Part model, mm, in its own coordinate system. Face numbers are marked on the shaded views. A direction names the side the tool comes from. Coordinates: 2 decimals unless noted, no trailing zeros. Write each loop counter-clockwise with the first axis right and the second up, starting at its lowest first coordinate (ties: lowest second). Pieces come first, ordered by that corner, then holes. Notation, with made-up numbers: (-25, 25) -> (29, 25) arc R16 cw to (29, 45) -> close; hole circle Ø5 at (57, -5.75). An arc over 180 degrees is marked (long way). One line per question, with ' | ' between items. Start each with the question number.
Item 1: Two-plate mould, pull along Y, no slides. Class the marked faces 1, 2 and 3: pulls with the +Y half, pulls with the -Y half, needs draft (parallel to the pull), parting line crosses it, or undercut.
Item 2: Probe probe 1 along Y at (x, z) = (0, -18); probe 2 along Z at (x, y) = (-20, 8.5). List the from-to ranges inside material, lowest first. Write a range as [from, to].
Item 3: Saw through at C-C (x = -43). List the corners of the cut face in (y, z), and give its area (3 significant figures).
Item 4: Saw through at B-B (y = 18). List the corners of the cut face in (x, z).
Item 5: 3-axis set-ups, long thin cutter, end or side, ignore diameter. For the marked faces 4 and 5: which of +Z, -Z, +X, -X, +Y, -Y reach the whole face in a straight line?
Item 6: Pin check, flat tips, straight feed: pin 1 (2 mm diameter, centred on x = 21.5, y = -9, fed in from -Z); pin 2 (5 mm diameter, centred on x = 0, y = 0, fed in from +Z). Stop position of each tip, or through.
Item 7: Saw through at A-A (z = -12). List the corners of the cut face in (x, y), and give its area (3 significant figures).
from build123d import *

# Parameters (mm, degrees)
F1_DEPTH = 10
F2_R     = 2
F3_DEPTH = 10
F2_R_2   = 4
F4_DEPTH = 5
F5_R     = 4.99999
F6_R     = 5
F6_R_2   = 2
F7_DEPTH = 25


# Not quite as in the source:
# - a fillet or chamfer is up to 0.001 mm smaller than in the source, because OpenCascade refuses the exact size


with BuildPart() as f1:
    # F0 (on Top) → F1 (new body)
    with BuildSketch(Plane.XY):
        with BuildLine():
            ThreePointArc((-50, -5), (-18.1801948466, -18.1801948466), (-5, -50))
            Line((-5, -50), (5, -50))
            ThreePointArc((5, -50), (18.1801948466, -18.1801948466), (50, -5))
            Line((50, -5), (50, 5))
            ThreePointArc((50, 5), (18.1801948466, 18.1801948466), (5, 50))
            Line((5, 50), (-5, 50))
            ThreePointArc((-5, 50), (-18.1801948466, 18.1801948466), (-50, 5))
            Line((-50, 5), (-50, -5))
        make_face()
    extrude(amount=F1_DEPTH)

    # F2 (on face) → F3 (cut, through all)
    with BuildSketch(Plane.XY.offset(10)):
        Circle(F2_R)
    extrude(amount=-F3_DEPTH, mode=Mode.SUBTRACT)

    # F2 (on face) → F4 (cut)
    with BuildSketch(Plane.XY.offset(10)):
        Circle(F2_R_2)
        Circle(F2_R, mode=Mode.SUBTRACT)
    extrude(amount=-F4_DEPTH, mode=Mode.SUBTRACT)

    # F5 (radius 5 in the source; OpenCascade refuses exactly that, so slightly less here)
    f5_edges = [f1.edges().sort_by_distance(p)[0] for p in [
        (5, 50, 5),
        (-5, 50, 5),
        (0, 50, 0),
        (0, 50, 10),
        (-50, 5, 5),
        (-50, -5, 5),
        (-50, 0, 0),
        (-50, 0, 10),
        (-5, -50, 5),
        (5, -50, 5),
        (0, -50, 0),
        (0, -50, 10),
        (50, -5, 5),
        (50, 5, 5),
        (50, 0, 0),
        (50, 0, 10),
    ]]
    fillet(f5_edges, radius=F5_R)

    # F6 (on face) → F7 (join)
    with BuildSketch(Plane(origin=(0, 0, 0), x_dir=(1, 0, 0), z_dir=(0, 0, -1))):
        Circle(F6_R)
        Circle(F6_R_2, mode=Mode.SUBTRACT)
    extrude(amount=F7_DEPTH)


solid = f1.part
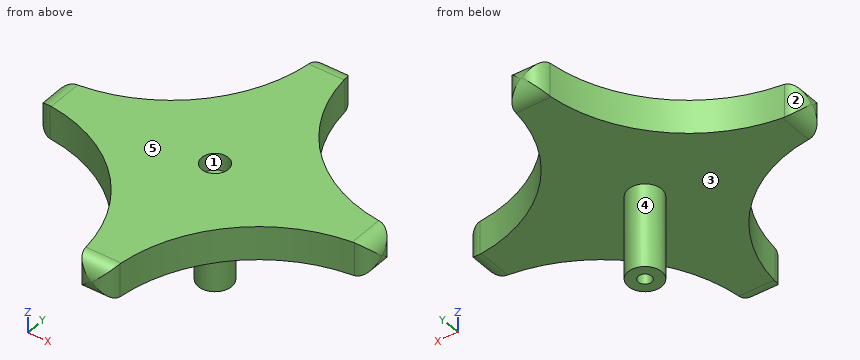
From the geometry:
1) face 1: undercut | face 2: pulls with the +Y half | face 3: needs draft
2) probe 1: [-5, -2], [2, 5] | probe 2: [0, 10]
3) outline: (-5.55, 0) -> (5.55, 0) -> (5.55, 10) -> (-5.55, 10) -> close | area: 111 mm2
4) outline: (-18.36, 0) -> (18.36, 0) -> (18.36, 10) -> (-18.36, 10) -> close
5) face 4: -Z | face 5: +Z, +X, -X, +Y, -Y
6) pin 1: z = 0 | pin 2: z = 5
7) outline: circle Ø10 at (0, 0); hole circle Ø4 at (0, 0) | area: 66.0 mm2
